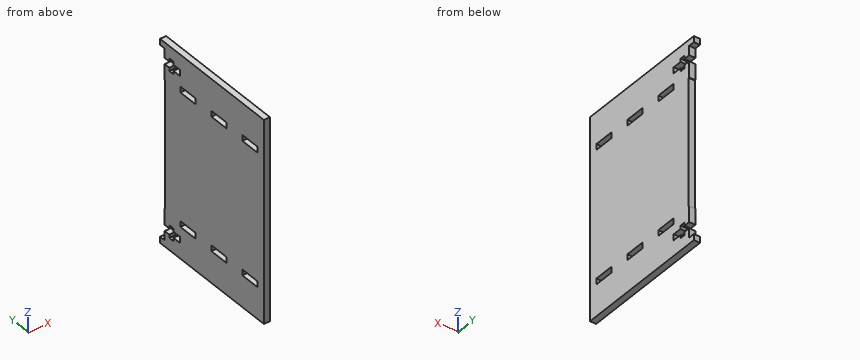
```python
from build123d import *

# Parameters (mm, degrees)
SKETCH1_W           = 100
SKETCH1_H           = 64
BOSS_EXTRUDE1_DEPTH = 3
SKETCH2_W           = 2.9
SKETCH2_H           = 9.8
CUT_EXTRUDE1_DEPTH  = 3
CUT_EXTRUDE2_DEPTH  = 10
SKETCH5_W           = 63
SKETCH5_H           = 0.35
CUT_EXTRUDE3_DEPTH  = 10
SKETCH6_W           = 3
SKETCH6_H           = 3
BOSS_EXTRUDE3_DEPTH = 3


with BuildPart() as part:
    # Sketch1 → Boss-Extrude1 (new body)
    with BuildSketch(Plane(origin=(0, 0, 0), x_dir=(0, 0, -1), z_dir=(1, 0, 0))):
        Rectangle(SKETCH1_W, SKETCH1_H)
    extrude(amount=BOSS_EXTRUDE1_DEPTH)

    # Sketch2 → Cut-Extrude1 (cut)
    with BuildSketch(Plane(origin=(3, 0, 0), x_dir=(0, 0, -1), z_dir=(1, 0, 0))):
        with Locations((-32.95, 17)):
            Rectangle(SKETCH2_W, SKETCH2_H)
        with Locations((-32.95, -3)):
            Rectangle(SKETCH2_W, SKETCH2_H)
        with Locations((-32.95, -23)):
            Rectangle(SKETCH2_W, SKETCH2_H)
        with Locations((32.95, -23)):
            Rectangle(SKETCH2_W, SKETCH2_H)
        with Locations((32.95, -3)):
            Rectangle(SKETCH2_W, SKETCH2_H)
        with Locations((32.95, 17)):
            Rectangle(SKETCH2_W, SKETCH2_H)
    extrude(amount=-CUT_EXTRUDE1_DEPTH, mode=Mode.SUBTRACT)

    # Sketch3 → Cut-Extrude2 (cut)
    with BuildSketch(Plane(origin=(3, 0, 0), x_dir=(0, 0, -1), z_dir=(1, 0, 0))):
        Polygon((-42.4, 32), (-42.4, 29), (-44, 29), (-44, 26.4), (-42.4, 26.4), (-42.4, 22), (-39.4, 22), (-39.4, 26.4), (-37.8, 26.4), (-37.8, 29), (-39.4, 29), (-39.4, 32), align=None)
    cut_extrude2 = extrude(amount=-CUT_EXTRUDE2_DEPTH, mode=Mode.SUBTRACT)

    # Mirror1: Cut-Extrude2 across plane
    add(cut_extrude2.mirror(Plane.XY), mode=Mode.SUBTRACT)

    # Sketch5 → Cut-Extrude3 (cut)
    with BuildSketch(Plane(origin=(3, 0, 0), x_dir=(0, 0, -1), z_dir=(1, 0, 0))):
        with Locations((0, 31.825)):
            Rectangle(SKETCH5_W, SKETCH5_H)
    extrude(amount=-CUT_EXTRUDE3_DEPTH, mode=Mode.SUBTRACT)

    # Sketch6 → Boss-Extrude3 (add)
    with BuildSketch(Plane.ZY):
        with Locations((-48.5, 33.5)):
            Rectangle(SKETCH6_W, SKETCH6_H)
        with Locations((48.5, 33.5)):
            Rectangle(SKETCH6_W, SKETCH6_H)
    extrude(amount=-BOSS_EXTRUDE3_DEPTH)


solid = part.part
```
Work out the finished part from the listing and answer in its coordinate system (mm). Round coordinates to 2 decimals unless told otherwise and drop trailing zeros. Loops run counter-clockwise (first coordinate to the right, second up) from the corner with the lowest first, then second, coordinate; pieces in that order, holes last. Notation, with made-up numbers: M 26.25,74.5 L 84.25,74.5 A25 ccw 84.25,87.5 Z; hole C -16.75,18.5 d4. An arc over 180 degrees is marked long. Use CSV: the item, a comma, the result in double quotes.
Q1. Section A-A, the plane y = -25 is taken. Determine the outline of the cut face in (x, z), then the cut area to 3 significant figures.
Determined:
outline,"M 0,-50 L 3,-50 L 3,-34.4 L 0,-34.4 Z; M 0,-31.5 L 3,-31.5 L 3,31.5 L 0,31.5 Z; M 0,34.4 L 3,34.4 L 3,50 L 0,50 Z"
area,"283 mm2"
Q2. This flat-tipped pin is pushed along its axis until it touches: pin 1 (0.5 mm diameter, centred on x = 1, z = -43, fed in from +Y). Where does it stop, or does it pass through?
Determined:
pin 1,"y = 32"
Q3. Consider L1, parallel to Z at x = 1.3, y = -21; L2, parallel to Y at x = 2.2, z = -33; L3, parallel to Y at x = 2.3, z = -38. Determine where each line is inside the solid, lowest interval first.
Determined:
L1,"-50 to -34.4, -31.5 to 31.5, 34.4 to 50"
L2,"-32 to -27.9, -18.1 to -7.9, 1.9 to 12.1, 21.9 to 32"
L3,"-32 to 26.4, 29 to 32"
Q4. Section B-B, the plane x = 1.15 is taken. State how many separate pieces and enclosed holes the cut face has, then the cut area to 3 significant figures.
Determined:
separate pieces,"1"
enclosed holes,"6"
area,"6,150 mm2"
Q5. Section C-C, the plane z = 8 is taken. Determine the outline of the cut face in (x, y).
Determined:
outline,"M 0,-32 L 3,-32 L 3,31.65 L 0,31.65 Z"
